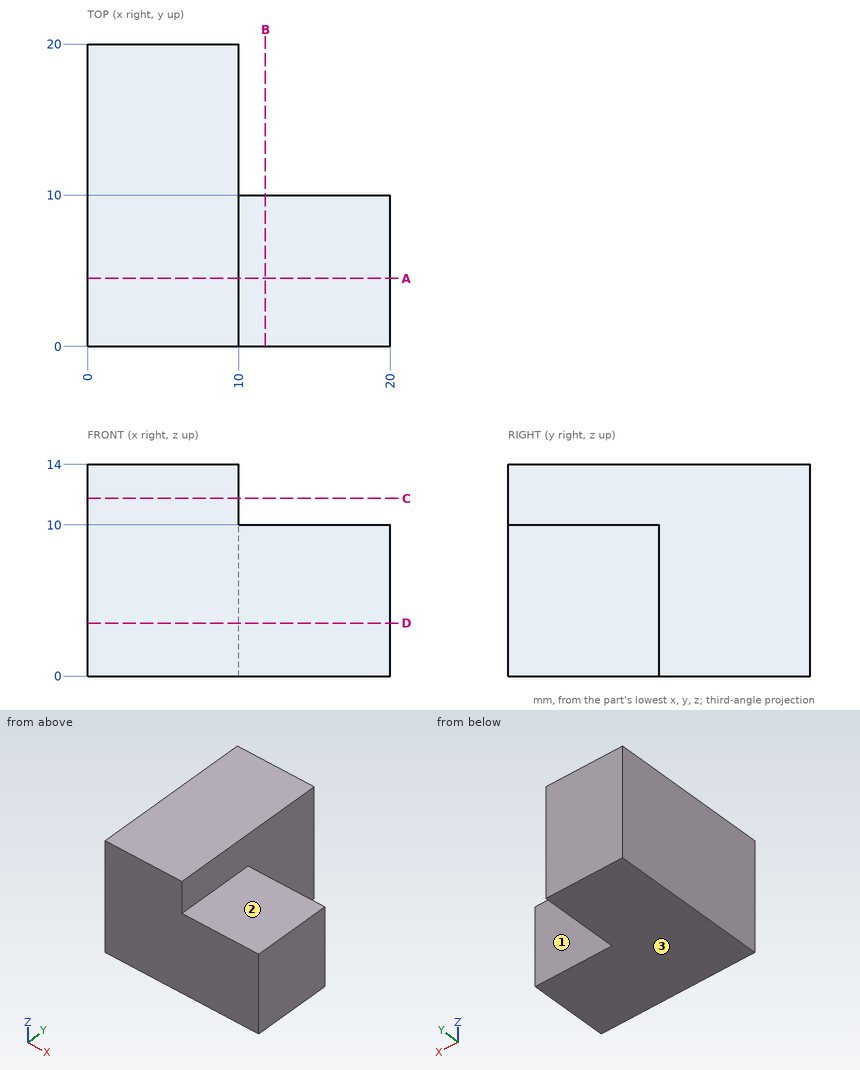
Design review of the part shown in the three views and the two pictorial views. Dimensions are in mm from the part's minimum x, y and z. A direction names the side the tool comes from. Give positions to 0.01 mm unless a question says otherwise; leave off trailing zeros. Order: outer loops, then holes, each group sorted by start corner. A loop starts at its lowest first (then second) coordinate and runs counter-clockwise, first axis right, second up. Notation, with made-up numbers: M -24.75,25 L 4.25,25 A31 cw 4.25,55 Z; hole C 84,37.25 d1. An arc over 180 degrees is marked long. Answer in a Markdown table with one row per item. Add a question column.
(1) Wall thickness on probe 1 along Z at (x, y) = (11.5, 7.5): over which ranges is the line inside the solid? List them lowest first. Write a range as [from, to].
(2) Consider section C-C on z = 11.75. State the section outline as (x, y) points, and give its area (3 significant figures).
(3) Consider section A-A on y = 4.5. State the section outline as (x, z) points.
(4) Consider section D-D on z = 3.5. State the section outline as (x, y) points, and give its area (3 significant figures).
(5) For pin 1 (3 mm diameter, centred on x = 14.5, y = 6, fed in from +Z); pin 2 (1 mm diameter, centred on y = 17, z = 3, fed in from +X); pin 3 (3 mm diameter, centred on x = 17.5, z = 5, fed in from +Y), all flat-tipped, find the tip position at first contact; note any pin that passes through.
(6) Consider section B-B on x = 11.75. State the section outline as (y, z) points, and give its area (3 significant figures).
(7) For the marked faces 1, 2 and 3, list the 3-axis set-ups (+Z, -Z, +X, -X, +Y, -Y) from which the entire face can be reached by the end or side of a thin tool; tool diameter is ignored.
Evaluation:
| question | item | result |
|---|---|---|
| 1 | probe 1 | z = [0, 10] |
| 2 | outline | M 0,0 L 10,0 L 10,20 L 0,20 Z |
| 2 | area | 200 mm^2 |
| 3 | outline | M 0,0 L 20,0 L 20,10 L 10,10 L 10,14 L 0,14 Z |
| 4 | outline | M 0,0 L 20,0 L 20,10 L 10,10 L 10,20 L 0,20 Z |
| 4 | area | 300 mm^2 |
| 5 | pin 1 | stops at z = 10 |
| 5 | pin 2 | stops at x = 10 |
| 5 | pin 3 | stops at y = 10 |
| 6 | outline | M 0,0 L 10,0 L 10,10 L 0,10 Z |
| 6 | area | 100 mm^2 |
| 7 | face 1 | +Z, -Z, +X, +Y |
| 7 | face 2 | +Z, +X, +Y, -Y |
| 7 | face 3 | -Z, +X, -X, +Y, -Y |
